from build123d import *

# Parameters (mm, degrees)
PAD_DEPTH    = 9.8
FILLET_R     = 0.25
SKETCH001_R  = 2.1
POCKET_DEPTH = 4.451
CHAMFER_SIZE = 0.5


with BuildPart() as part:
    # Sketch → Pad (new body)
    with BuildSketch(Plane.XY):
        with BuildLine():
            Line((-5.2, 0), (-2.95, 0))
            Line((-2.95, 0), (-2.95, -1.2))
            Line((-2.95, -1.2), (2.95, -1.2))
            Line((2.95, -1.2), (2.95, 0))
            Line((2.95, 0), (5.2, 0))
            ThreePointArc((5.2, 0), (5.477926, 0.187053), (5.409273, 0.514953))
            Line((2.6, 3.25), (5.409273, 0.514953))
            Line((-2.6, 3.25), (2.6, 3.25))
            Line((-5.409273, 0.514953), (-2.6, 3.25))
            ThreePointArc((-5.409273, 0.514953), (-5.477926, 0.187053), (-5.2, 0))
        make_face()
    extrude(amount=PAD_DEPTH)

    # Fillet
    fillet_edges = [part.edges().sort_by_distance(p)[0] for p in [
        (2.95, 0, 4.9),
        (2.95, -1.2, 4.9),
        (-2.95, -1.2, 4.9),
        (-2.95, 0, 4.9),
        (-2.6, 3.25, 4.9),
        (2.6, 3.25, 4.9),
    ]]
    fillet(fillet_edges, radius=FILLET_R)

    # Sketch001 (on Face10 of Fillet) → Pocket (cut, through all)
    with BuildSketch(Plane.XZ.offset(1.2)):
        with Locations((0, 4.5)):
            Circle(SKETCH001_R)
    extrude(amount=-POCKET_DEPTH, mode=Mode.SUBTRACT)

    # Chamfer
    chamfer_edges = [part.edges().sort_by_distance(p)[0] for p in [
        (-2.1, -1.2, 4.5),
        (2.1, 1.025, 4.5),
        (-2.1, 3.25, 4.5),
    ]]
    chamfer(chamfer_edges, length=CHAMFER_SIZE)


solid = part.part
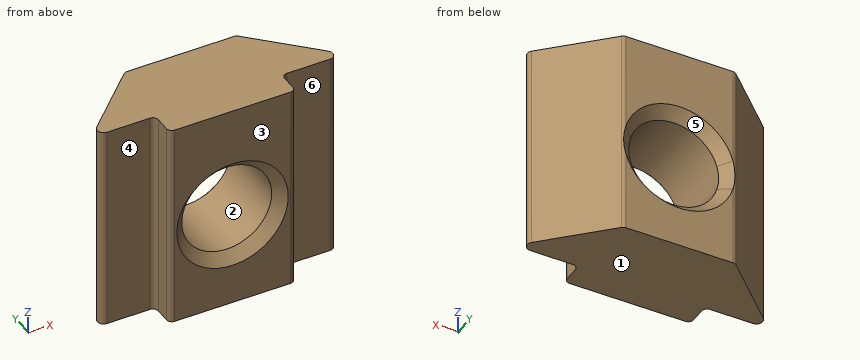
Could you check a few things on this model? Use its own coordinates, in mm. Face numbers are marked on the shaded views. A direction names the side the tool comes from. Round coordinates to 2 decimals unless told otherwise and drop trailing zeros. Order: outer loops, then holes, each group sorted by start corner. A loop starts at its lowest first (then second) coordinate and runs counter-clockwise, first axis right, second up.
Q1. Imagine slicing it at D-D, the plane x = 4. List the corners of the cut face in (y, z) for me.
Geometry says:
outline: (0, 0) - (1.89, 0) - (1.89, 9.8) - (0, 9.8) - close
Q2. I'm going to push flat-ended pins straight in: P1, Ø1, axis at x = 4.5, z = 7, coming from the -Y side; P2, Ø1, axis at x = 4, z = 7, coming from the +Y side. Where does each tip first touch, or does it pass through?
Geometry says:
P1: stops at y = 0
P2: stops at y = 2.37
Q3. Imagine slicing it at B-B, the plane z = 8. List the corners of the cut face in (x, y) for me.
Geometry says:
outline: (-5.41, 0.51) arc R0.3 ccw to (-5.2, 0) - (-3.2, 0) arc R0.25 cw to (-2.95, -0.25) - (-2.95, -0.95) arc R0.25 ccw to (-2.7, -1.2) - (2.7, -1.2) arc R0.25 ccw to (2.95, -0.95) - (2.95, -0.25) arc R0.25 cw to (3.2, 0) - (5.2, 0) arc R0.3 ccw to (5.41, 0.51) - (2.67, 3.18) arc R0.25 ccw to (2.5, 3.25) - (-2.5, 3.25) arc R0.25 ccw to (-2.67, 3.18) - close
Q4. Thinking about a two-plate mould opening in Z: for the marked faces 1, 2 and 3, which applies, released by +Z, released by -Z, zero draft, split by the parting line, or undercut?
Geometry says:
face 1: released by -Z
face 2: undercut
face 3: zero draft
Q5. Imagine slicing it at A-A, the plane x = 0. List the corners of the cut face in (y, z) for me.
Geometry says:
outline: (-1.2, 0) - (3.25, 0) - (3.25, 1.9) - (2.75, 2.4) - (-0.7, 2.4) - (-1.2, 1.9) - close; (-1.2, 7.1) - (-0.7, 6.6) - (2.75, 6.6) - (3.25, 7.1) - (3.25, 9.8) - (-1.2, 9.8) - close
Q6. Please list where these lines run through material, in increasing order: probe 1 along Z at (x, y) = (0, 1.5); probe 2 along X at (y, z) = (-0.4, 4.75); probe 3 along X at (y, z) = (0.9, 4.5).
Geometry says:
probe 1: z = 0 to 2.4, 6.6 to 9.8
probe 2: x = -2.95 to -2.09, 2.09 to 2.95
probe 3: x = -5.01 to -2.1, 2.1 to 5.01
Q7. Imagine slicing it at C-C, the plane y = 1.4. List the corners of the cut face in (x, z) for me, then the cut area to 3 significant figures.
Geometry says:
outline: (-4.5, 0) - (4.5, 0) - (4.5, 9.8) - (-4.5, 9.8) - close; hole circle Ø4.2 at (0, 4.5)
area: 74.3 mm2
Q8. Which directions (+Z, -Z, +X, -X, +Y, -Y) give clear straight access to the entire face, cutting with the end or side of a thin tool? Please do the marked faces 4, 5 and 6.
Geometry says:
face 4: +Z, -Z, -X, -Y
face 5: +Y
face 6: +Z, -Z, +X, -Y
